Source: three-view drawing plus pictorial views. Frame: mm from the lowest corner of the part. A direction names the side the tool comes from. Round coordinates to 2 decimals unless told otherwise and drop trailing zeros. Write each loop counter-clockwise with the first axis right and the second up, starting at its lowest first coordinate (ties: lowest second). Pieces come first, ordered by that corner, then holes. Notation, with made-up numbers: (-6.75, -14.75) -> (16.25, -14.75) arc R16 cw to (16.25, -5.75) -> close; hole circle Ø10 at (-12, 16). An arc over 180 degrees is marked (long way). Put each result on its own line as item: value.
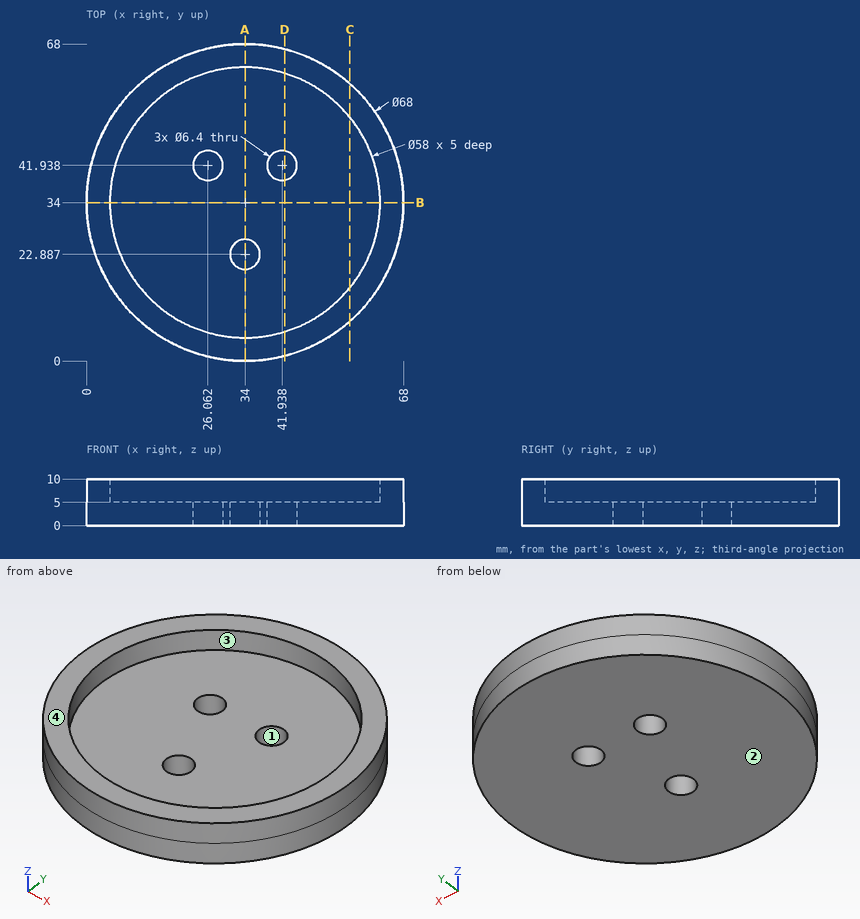
Q1. Cut plane D-D on x = 42.5. Output: boundary loops of the cut face in (y, z).
Ans:
outline: (1.08, 0) -> (38.79, 0) -> (38.79, 5) -> (6.27, 5) -> (6.27, 10) -> (1.08, 10) -> close; (45.09, 0) -> (66.92, 0) -> (66.92, 10) -> (61.73, 10) -> (61.73, 5) -> (45.09, 5) -> close
Q2. Pin query (flat end, axial travel): pin 1 (4 mm diameter, centred on y = 35.5, z = 8.5, fed in from +X); pin 2 (1 mm diameter, centred on x = 13, z = 4.5, fed in from -Y) (1 decimal); pin 3 (10 mm diameter, centred on x = 34, y = 22.89, fed in from +Z); pin 4 (6 mm diameter, centred on y = 51.5, z = 2.5, fed in from +X). Return the tip coordinate at first contact, or that it passes through.
Ans:
pin 1: stops at x = 68
pin 2: stops at y = 6.9
pin 3: stops at z = 5
pin 4: stops at x = 64.75
Q3. Cut plane C-C on x = 56.5. Output: boundary loops of the cut face in (y, z), and give its area (3 significant figures).
Ans:
outline: (8.51, 0) -> (59.49, 0) -> (59.49, 10) -> (52.3, 10) -> (52.3, 5) -> (15.7, 5) -> (15.7, 10) -> (8.51, 10) -> close
area: 327 mm^2
Q4. Cut plane A-A on x = 34. Output: boundary loops of the cut face in (y, z).
Ans:
outline: (0, 0) -> (19.69, 0) -> (19.69, 5) -> (5, 5) -> (5, 10) -> (0, 10) -> close; (26.09, 0) -> (68, 0) -> (68, 10) -> (63, 10) -> (63, 5) -> (26.09, 5) -> close
Q5. Material intervals for line 1 (Y direction, x = 34, z = 7.5); line 2 (Z direction, x = 29, y = 21.5); line 3 (Y direction, x = 26.5, z = 9), sorted ascending. Write a range as [from, to].
Ans:
line 1: y = [0, 5], [63, 68]
line 2: z = [0, 5]
line 3: y = [0.84, 5.99], [62.01, 67.16]
Q6. Reachability of the marked faces 3 and 4 from +Z, -Z, +X, -X, +Y, -Y: full face, straight path, thin tool, end or side. Return the list, or none.
Ans:
face 3: +Z
face 4: +Z, +X, -X, +Y, -Y
Q7. Draft query along Y for the marked faces 1 and 2. Return one class per face: +Y half, -Y half, draft (parallel to the pull), parting line (faces both ways), or undercut.
Ans:
face 1: undercut
face 2: draft
Q8. Cut plane B-B on y = 34. Output: boundary loops of the cut face in (x, z).
Ans:
outline: (0, 0) -> (68, 0) -> (68, 10) -> (63, 10) -> (63, 5) -> (5, 5) -> (5, 10) -> (0, 10) -> close
